Part model, mm, in its own coordinate system. Face numbers are marked on the shaded views. A direction names the side the tool comes from. Give positions to 0.01 mm unless a question says otherwise; leave off trailing zeros. Write each loop counter-clockwise with the first axis right and the second up, starting at its lowest first coordinate (ties: lowest second). Pieces come first, ordered by that corner, then holes.
from build123d import *

# Parameters (mm, degrees)
F0_R     = 12.5
F1_DEPTH = 25
F3_DEPTH = 25


with BuildPart() as f1:
    # F0 (on Top) → F1 (new body)
    with BuildSketch(Plane.XY):
        with BuildLine():
            Line((-6, 28.747727), (-6, 13.747727))
            ThreePointArc((-6, 13.747727), (-12.990381, 7.5), (-14.905881, -1.677711))
            Line((-14.905881, -1.677711), (-27.896262, -9.177711))
            Line((-27.896262, -9.177711), (-24.896262, -14.373864))
            Line((-24.896262, -14.373864), (-21.896262, -19.570016))
            Line((-21.896262, -19.570016), (-8.905881, -12.070016))
            ThreePointArc((-8.905881, -12.070016), (0, -15), (8.905881, -12.070016))
            Line((8.905881, -12.070016), (21.896262, -19.570016))
            Line((21.896262, -19.570016), (24.896262, -14.373864))
            Line((24.896262, -14.373864), (27.896262, -9.177711))
            Line((27.896262, -9.177711), (14.905881, -1.677711))
            ThreePointArc((14.905881, -1.677711), (12.990381, 7.5), (6, 13.747727))
            Line((6, 13.747727), (6, 28.747727))
            Line((6, 28.747727), (0, 28.747727))
            Line((0, 28.747727), (-6, 28.747727))
        make_face()
        Circle(F0_R, mode=Mode.SUBTRACT)
    extrude(amount=F1_DEPTH)

    # F2 (on face) → F3 (cut)
    with BuildSketch(Plane.XY.offset(25)):
        with BuildLine():
            Line((4.5, 28.747727), (-4.5, 28.747727))
            Line((-4.5, 28.747727), (-4.5, 14.309088))
            ThreePointArc((-4.5, 14.309088), (0, 15), (4.5, 14.309088))
            Line((4.5, 14.309088), (4.5, 28.747727))
        make_face()
        with BuildLine():
            Line((27.146262, -10.476749), (14.642034, -3.25743))
            ThreePointArc((14.642034, -3.25743), (12.990381, -7.5), (10.142034, -11.051658))
            Line((10.142034, -11.051658), (22.646262, -18.270978))
            Line((22.646262, -18.270978), (27.146262, -10.476749))
        make_face()
        with BuildLine():
            Line((-22.646262, -18.270978), (-10.142034, -11.051658))
            ThreePointArc((-10.142034, -11.051658), (-12.990381, -7.5), (-14.642034, -3.25743))
            Line((-14.642034, -3.25743), (-27.146262, -10.476749))
            Line((-27.146262, -10.476749), (-22.646262, -18.270978))
        make_face()
    extrude(amount=-F3_DEPTH, mode=Mode.SUBTRACT)


solid = f1.part
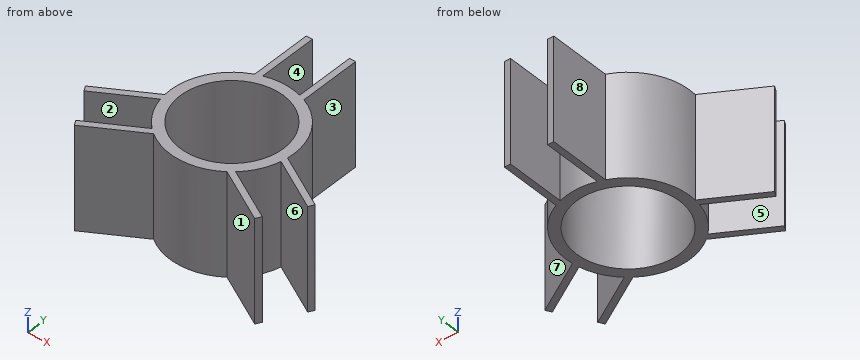
1) 3-axis set-ups, long thin cutter, end or side, ignore diameter. For the marked faces 1, 2, 3, 4 and 5: which of +Z, -Z, +X, -X, +Y, -Y reach the whole face in a straight line?
Check result:
face 1: +Z, -Z, -Y
face 2: +Z, -Z
face 3: +Z, -Z, +X, +Y
face 4: +Z, -Z, +Y
face 5: +Z, -Z, -X
2) Saw through at C-C (y = -13.5). Write the cut outline in (x, z), and give its area (3 significant figures).
Check result:
outline: (-14.38, 0) - (-11.38, 0) - (-11.38, 25) - (-14.38, 25) - close; (-6.54, 0) - (6.54, 0) - (6.54, 25) - (-6.54, 25) - close; (11.38, 0) - (14.38, 0) - (14.38, 25) - (11.38, 25) - close
area: 477 mm2
3) Mould opens along X. For the marked faces 6, 7 and 8 say: +X half, -X half, draft (parallel to the pull), parting line (faces both ways), or undercut.
Check result:
face 6: undercut
face 7: +X half
face 8: -X half
4) Saw through at A-A (x = 0). Write the cut outline in (y, z), and give its area (3 significant figures).
Check result:
outline: (-15, 0) - (-12.5, 0) - (-12.5, 25) - (-15, 25) - close; (12.5, 0) - (15, 0) - (15, 25) - (12.5, 25) - close
area: 125 mm2
5) Saw through at B-B (y = 24.5). Write the cut outline in (x, z).
Check result:
outline: (-6, 0) - (-4.5, 0) - (-4.5, 25) - (-6, 25) - close; (4.5, 0) - (6, 0) - (6, 25) - (4.5, 25) - close
6) Flat gauge pins, fed straight in: P1, Ø7, axis at y = 21, z = 10.5, coming from the -X side; P2, Ø1.5, axis at x = 3, z = 10.5, coming from the +Y side; P3, Ø1.5, axis at y = 4.5, z = 22, coming from the +X side. Where does each tip first touch, or does it go through?
Check result:
P1: stops at x = -6
P2: stops at y = 14.83
P3: stops at x = 14.52
7) Drill centre lines: L1, parallel to X at y = 20, z = 24.25; L2, parallel to X at y = -5, z = 21; L3, parallel to Y at x = 0.5, z = 22.5. Where is each one in solid material? Low to high.
Check result:
L1: x = -6 to -4.5, 4.5 to 6
L2: x = -20.66 to -17.66, -14.14 to -11.46, 11.46 to 14.14, 17.66 to 20.66
L3: y = -14.99 to -12.49, 12.49 to 14.99
